Autodesk Inventor part; units mm, degrees
ref_plane "Start Plane" through (0, 0, -11.547) normal (0, 0, 1) x (1, 0, 0)
ref_plane "End Plane" through (0, 0, 704.3673) normal (0, 0, 1) x (1, 0, 0)
ref_plane "Work Plane4" through (-20, 0, -11.547) normal (0.5, 0, -0.866) x (-0.866, 0, -0.5)
ref_plane "Start Plane" through (0, 0, -11.547) normal (0, 0, 1) x (1, 0, 0)
ref_plane "End Plane" through (0, 0, 704.3673) normal (0, 0, 1) x (1, 0, 0)
sketch "Sketch" plane through (0, 0, 0) normal (0, 0, 1) x (1, 0, 0)
  line L0 (-20, -16) -> (-20, 16)
  line L1 (-16, 20) -> (16, 20)
  line L2 (20, 16) -> (20, -16)
  line L3 (16, -20) -> (-16, -20)
  arc A0 (-20, -16) -> (-16, -20) centre (-16, -16) ccw
  arc A1 (20, 16) -> (16, 20) centre (16, 16) ccw
  arc A2 (-16, 20) -> (-20, 16) centre (-16, 16) ccw
  arc A3 (16, -20) -> (20, -16) centre (16, -16) ccw
  arc A4 (-16, 18) -> (-18, 16) centre (-16, 16) ccw
  line L4 (-16, 18) -> (16, 18)
  arc A5 (18, 16) -> (16, 18) centre (16, 16) ccw
  line L5 (18, 16) -> (18, -16)
  arc A6 (16, -18) -> (18, -16) centre (16, -16) ccw
  line L6 (16, -18) -> (-16, -18)
  arc A7 (-18, -16) -> (-16, -18) centre (-16, -16) ccw
  line L7 (-18, -16) -> (-18, 16)
  line L8 (0, 29.1598) -> (0, -29.1598) construction
  line L9 (-29.1598, 0) -> (29.1598, 0) construction
  dimension "d7" = 4
  dimension "d9" = 40
  dimension "d11" = 40
  dimension "d12" = 2
  dimension "d15" = 20
  dimension "d16" = 20
extrude "Body" add sketch "Sketch" along normal up to surface (715.9143 mm away) from surface at -11.547
sketch "Sketch3" plane through (0, 0, 0) normal (0, 0, 1) x (1, 0, 0)
  line L0 (0, 0) -> (10, 0)
ref_plane "Work Plane3" through (0, 0, 0) normal (0, -1, 0) x (1, 0, 0)
sketch "Sketch4" plane through (0, 0, 0) normal (0, -1, 0) x (1, 0, 0)
  line L0 (-2, -11.547) -> (12, -11.547)
  line L1 (-2, 704.3673) -> (12, 704.3673)
  dimension "d18" = 715.9143
ref_plane "Work Plane4" through (-20, 0, -11.547) normal (0.5, 0, -0.866) x (-0.866, 0, -0.5)
split "Split1" plane through (-20, 0, -11.547) removes the side toward (0.5, 0, -0.866)
ref_plane "Work Plane5" through (-20, 0, 704.3673) normal (0.5, 0, 0.866) x (0.866, 0, -0.5)
split "Split2" plane through (-20, 0, 704.3673) removes the side toward (0.5, 0, 0.866)
equation "\"d7\" = G_IR"
equation "\"d9\" = G_W"
equation "\"d11\" = G_H"
equation "\"d12\" = G_T"
equation "\"d15\" = 0.5 * d9"
equation "\"d16\" = 0.5 * d11"
equation "\"d3\" = G_L"
equation "\"G_W\" = 40"
equation "\"G_H\" = 40"
equation "\"G_T\" = 2"
equation "\"G_IR\" = 4"
equation "\"G_L\" = d18"
equation "\"G_OFFSET_START\" = 11.54701"
equation "\"G_OFFSET_END\" = 11.54701"
equation "\"d13\" = -G_OFFSET_START"
equation "\"d14\" = G_OFFSET_END + B_L"
equation "\"B_L\" = 692.82032"
properties part number "ISO 10799-2 - 40x40x2 - 715,91" material "Steel, Mild"
For this review, take the finished solid that the model builds, in its own axes (mm). A direction names the side the tool comes from. Round coordinates to 2 decimals unless told otherwise and drop trailing zeros. Write each loop counter-clockwise with the first axis right and the second up, starting at its lowest first coordinate (ties: lowest second). Pieces come first, ordered by that corner, then holes. Notation, with made-up numbers: (15.5, -29.75) - (32.5, -29.75) arc R13 cw to (32.5, -24.75) - close; hole circle Ø4 at (63.25, 85.25). An arc over 180 degrees is marked (long way). Answer as a JSON object with one key per item and string values.
1. To check wall thickness, follow line 1 along Y through (x, z) = (-9, 229); line 2 along X through (y, z) = (16.5, 381). State the ranges of each line that lie inside material, in increasing order.
Response values:
{"line 1": "y = -20 to -18, 18 to 20", "line 2": "x = -19.97 to -17.94, 17.94 to 19.97"}
2. Draft analysis for pull direction X (two halves, no side actions). For faces 3 (the face through (-0.09, -19.35, 692.87)), 4 (the face through (0, -20, 341)), 5 (the face through (-18, 0, 341)), state which applies: +X half, -X half, draft (parallel to the pull), parting line (faces both ways), or undercut.
Response values:
{"face 3": "+X half", "face 4": "draft", "face 5": "undercut"}
3. For pin 1 Ø2 at (x, y) = (0.5, 15.5) entering from -Z, flat-tipped, find the tip position at first contact; note if it passes through.
Response values:
{"pin 1": "passes through"}
4. We need section C-C on z = 41.5. Give the boundary of the cut face in (x, y), then the cut area to 3 significant figures.
Response values:
{"outline": "(-20, -16) arc R4 ccw to (-16, -20) - (16, -20) arc R4 ccw to (20, -16) - (20, 16) arc R4 ccw to (16, 20) - (-16, 20) arc R4 ccw to (-20, 16) - close; hole (-18, -16) arc R2 ccw to (-16, -18) - (16, -18) arc R2 ccw to (18, -16) - (18, 16) arc R2 ccw to (16, 18) - (-16, 18) arc R2 ccw to (-18, 16) - close", "area": "294 mm2"}
5. We need section A-A on y = -2.5. Give the boundary of the cut face in (x, z).
Response values:
{"outline": "(-20, -11.55) - (-18, -10.39) - (-18, 703.21) - (-20, 704.37) - close; (18, 10.39) - (20, 11.55) - (20, 681.27) - (18, 682.43) - close"}
6. Tool access review of faces 1 (the face through (0, 20, 341)), 2 (the face through (0, 18, 341)): name each direction out of +Z, -Z, +X, -X, +Y, -Y from which nothing blocks a thin tool from reaching the whole face with its end or side.
Response values:
{"face 1": "+Z, -Z, +X, -X, +Y", "face 2": "+Z, -Z"}
7. We need section B-B on x = -2.5. Give the boundary of the cut face in (y, z), then the cut area to 3 significant figures.
Response values:
{"outline": "(-20, -1.44) - (-18, -1.44) - (-18, 694.26) - (-20, 694.26) - close; (18, -1.44) - (20, -1.44) - (20, 694.26) - (18, 694.26) - close", "area": "2,780 mm2"}
